Job drawing, mm, ordinate dimensions from the low corner. One solid piece. A direction names the side the tool comes from. Give positions to 0.01 mm unless a question says otherwise; leave off trailing zeros. Loops run counter-clockwise (first coordinate to the right, second up) from the corner with the lowest first, then second, coordinate; pieces in that order, holes last. Notation, with made-up numbers: M 58.5,36.25 L 108.5,36.25 A13 cw 108.5,57.25 Z; hole C 79,88.5 d10. An arc over 180 degrees is marked long. Answer as CSV lines item,"result".
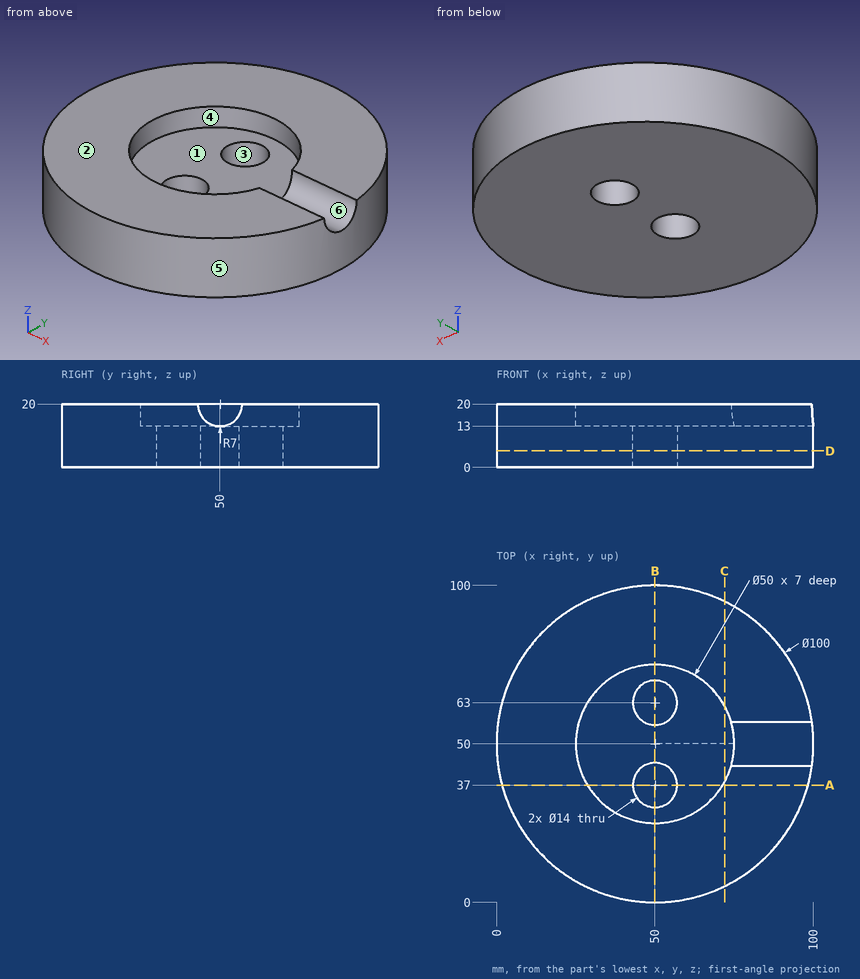
1) Flat gauge pins, fed straight in: pin 1 (10 mm diameter, centred on x = 26, z = 17, fed in from -Y); pin 2 (6 mm diameter, centred on y = 77.5, z = 18, fed in from +X); pin 3 (12 mm diameter, centred on y = 15.5, z = 8.5, fed in from -X); pin 4 (18 mm diameter, centred on x = 50, y = 63, fed in from -Z). Where does each tip first touch, or does it go through?
Answer below:
pin 1,"stops at y = 3.75"
pin 2,"stops at x = 93.59"
pin 3,"stops at x = 8.92"
pin 4,"stops at z = 0"
2) Band-saw the part on D-D on z = 5.25. Give the cut face in (x, y), and give its area (3 significant figures).
Answer below:
outline,"C 50,50 d100; hole C 50,37 d14; hole C 50,63 d14"
area,"7,550 mm^2"
3) Mould opens along X. For the marked faces 3, 4, 5 and 6 say: +X half, -X half, draft (parallel to the pull), parting line (faces both ways), or undercut.
Answer below:
face 3,"undercut"
face 4,"undercut"
face 5,"parting line"
face 6,"draft"
4) Drill centre lines: line 1 (Y direction, x = 50, z = 3.5); line 2 (Y direction, x = 50, z = 17.25); line 3 (Z direction, x = 33, y = 37). Where is each one in solid material? Low to high. Write a range as from..to.
Answer below:
line 1,"y = 0..30, 44..56, 70..100"
line 2,"y = 0..25, 75..100"
line 3,"z = 0..13"
5) Which spindle directions (+Z, -Z, +X, -X, +Y, -Y) get a long thin tool onto all of the face, cutting with end or side? Do the marked faces 1 and 2. Say none if no direction does.
Answer below:
face 1,"+Z"
face 2,"+Z, +X, -X, +Y, -Y"
6) Band-saw the part on A-A on y = 37. Give the cut face in (x, z), and give its area (3 significant figures).
Answer below:
outline,"M 1.72,0 L 43,0 L 43,13 L 28.65,13 L 28.65,20 L 1.72,20 Z; M 57,0 L 98.28,0 L 98.28,20 L 71.35,20 L 71.35,13 L 57,13 Z"
area,"1,450 mm^2"
7) Band-saw the part on C-C on x = 72. Give the cut face in (y, z), and give its area (3 significant figures).
Answer below:
outline,"M 5.1,0 L 94.9,0 L 94.9,20 L 61.87,20 L 61.87,13 L 38.13,13 L 38.13,20 L 5.1,20 Z"
area,"1,630 mm^2"
8) Band-saw the part on B-B on x = 50. Give the cut face in (y, z).
Answer below:
outline,"M 0,0 L 30,0 L 30,13 L 25,13 L 25,20 L 0,20 Z; M 44,0 L 56,0 L 56,13 L 44,13 Z; M 70,0 L 100,0 L 100,20 L 75,20 L 75,13 L 70,13 Z"
